Check sheet for the modelled part. Datum: model origin and axes. Units: mm. Coordinates: 2 decimals unless noted, no trailing zeros. Write each loop counter-clockwise with the first axis right and the second up, starting at its lowest first coordinate (ties: lowest second). Pieces come first, ordered by that corner, then holes. Notation, with made-up numbers: M 10,33 L 22,33 A16 cw 22,47 Z; hole C 49,73.5 d7. An arc over 180 degrees is marked long. Answer as CSV lines item,"result". Start each with the question number.
Q1. Sectioned sample at A-A, the plane y = 9.5. Record the cut outline in (x, z) (1 decimal).
Q2. Depth check by flat-ended pin: pin 1 Ø4.5 at (x, z) = (0, 57.15) entering from +Y; pin 2 Ø3 at (x, z) = (3.18, 394.88) entering from -Y; pin 3 Ø1.5 at (y, z) = (-20, 205) entering from +X. Enter the tip coordinate at first touch or a pass-through.
Q3. Thickness scan on line 1 along X through (y, z) = (-2, 87); line 2 along Y through (x, z) = (6, 346); line 3 along X through (y, z) = (-22, 296.5). Record the ranges inside material, lowest first. Write a range as from..to.
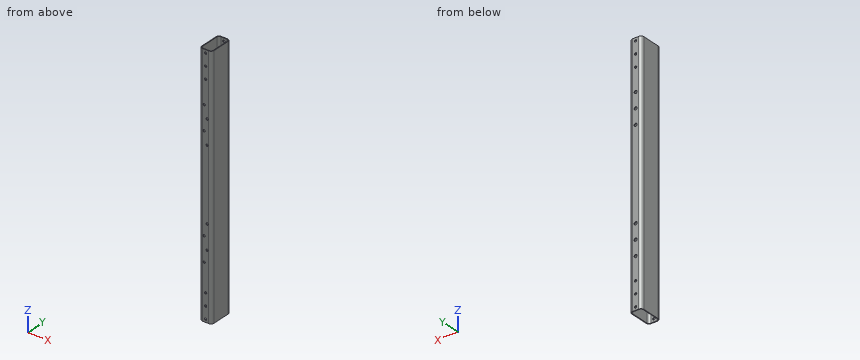
from build123d import *

# Parameters (mm, degrees)
EXTRUDE_THIN1_DEPTH               = 527.685
F_3_16_0_1875_DIAMETER_HOLE1_D    = 4.7625
F_3_16_0_195_DIAMETER_HOLE1_D     = 4.953
F_3_16_0_195_DIAMETER_HOLE1_DEPTH = 1.5875
F_1_4_0_25_DIAMETER_HOLE1_D       = 6.35
F_1_4_0_25_DIAMETER_HOLE1_DEPTH   = 25.4
F_1_4_0_25_DIAMETER_HOLE1_TIP     = 1.907732465


with BuildPart() as part:
    # Sketch1 → Extrude-Thin1 (new body)
    with BuildSketch(Plane.XY):
        with BuildLine():
            Line((-12.7, 19.05), (-12.7, -19.05))
            ThreePointArc((-12.7, -19.05), (-10.840128061, -23.540128061), (-6.35, -25.4))
            Line((-6.35, -25.4), (6.35, -25.4))
            ThreePointArc((6.35, -25.4), (10.840128061, -23.540128061), (12.7, -19.05))
            Line((12.7, -19.05), (12.7, 19.05))
            ThreePointArc((12.7, 19.05), (10.840128061, 23.540128061), (6.35, 25.4))
            Line((6.35, 25.4), (-6.35, 25.4))
            ThreePointArc((-6.35, 25.4), (-10.840128061, 23.540128061), (-12.7, 19.05))
        make_face()
        with BuildLine():
            Line((-11.1125, 19.05), (-11.1125, -19.05))
            ThreePointArc((-11.1125, -19.05), (-9.717596045, -22.417596045), (-6.35, -23.8125))
            Line((-6.35, -23.8125), (6.35, -23.8125))
            ThreePointArc((6.35, -23.8125), (9.717596045, -22.417596045), (11.1125, -19.05))
            Line((11.1125, -19.05), (11.1125, 19.05))
            ThreePointArc((11.1125, 19.05), (9.717596045, 22.417596045), (6.35, 23.8125))
            Line((6.35, 23.8125), (-6.35, 23.8125))
            ThreePointArc((-6.35, 23.8125), (-9.717596045, 22.417596045), (-11.1125, 19.05))
        make_face(mode=Mode.SUBTRACT)
    extrude(amount=EXTRUDE_THIN1_DEPTH)

    # 3/16 (0.1875) Diameter Hole1 (through all)
    with Locations(Plane(origin=(0, 25.4, 521.335), x_dir=(0, 0, 1), z_dir=(0, 1, 0))):
        with Locations((0, 0), (-514.985, 0), (-489.585, 0), (-464.185, 0), (-25.4, 0), (-50.8, 0)):
            Hole(F_3_16_0_1875_DIAMETER_HOLE1_D / 2)

    # 3/16 (0.195) Diameter Hole1
    with Locations(Plane(origin=(0, -25.4, 0), x_dir=(-1, 0, 0), z_dir=(0, -1, 0))):
        with Locations((3.175, -115.479743879), (-3.175, -140.879743879), (3.175, -166.279743879), (-3.175, -191.679743879), (-3.175, -344.079743879), (3.175, -369.479743879), (-3.175, -394.879743879), (3.175, -420.279743879)):
            Hole(F_3_16_0_195_DIAMETER_HOLE1_D / 2, depth=F_3_16_0_195_DIAMETER_HOLE1_DEPTH)

    # 1/4 (0.25) Diameter Hole1
    with Locations(Plane(origin=(0, 25.4, 0), x_dir=(1, 0, 0), z_dir=(0, 1, 0))):
        with Locations((0, -104.85), (0, -136.6), (0, -168.35), (0, -422.374806202), (0, -390.624806202), (0, -358.874806202)):
            Hole(F_1_4_0_25_DIAMETER_HOLE1_D / 2, depth=F_1_4_0_25_DIAMETER_HOLE1_DEPTH)
            with Locations((0, 0, -(F_1_4_0_25_DIAMETER_HOLE1_DEPTH + F_1_4_0_25_DIAMETER_HOLE1_TIP / 2))):  # 118° drill point
                Cone(0, F_1_4_0_25_DIAMETER_HOLE1_D / 2, F_1_4_0_25_DIAMETER_HOLE1_TIP, mode=Mode.SUBTRACT)


solid = part.part
Output:
1,outline,"M -12.7,0 L -11.1,0 L -11.1,527.7 L -12.7,527.7 Z; M 11.1,0 L 12.7,0 L 12.7,527.7 L 11.1,527.7 Z"
2,pin 1,"passes through"
2,pin 2,"stops at y = 23.81"
2,pin 3,"stops at x = 12.7"
3,line 1,"x = -12.7..-11.11, 11.11..12.7"
3,line 2,"y = -25.4..-23.81, 23.81..25.4"
3,line 3,"x = -11.97..-10.09, 10.09..11.97"
